Design review of the part built by this model. Coordinates are the model's own, in mm. A direction names the side the tool comes from. Coordinates: 2 decimals unless noted, no trailing zeros. Order: outer loops, then holes, each group sorted by start corner. A loop starts at its lowest first (then second) coordinate and runs counter-clockwise, first axis right, second up. Notation, with made-up numbers: M 82.5,15 L 101.5,15 A24 cw 101.5,25 Z; hole C -37,10.25 d7. An arc over 180 degrees is marked long. Answer as a JSON object with one key per item and string values.
Autodesk Inventor part; units mm, degrees
ref_plane "YZ Plane" through (0, 0, 0) normal (1, 0, 0) x (0, 1, 0)
ref_plane "XZ Plane" through (0, 0, 0) normal (0, 1, 0) x (-1, 0, 0)
ref_plane "XY Plane" through (0, 0, 0) normal (0, 0, 1) x (1, 0, 0)
sketch "Sketch1" plane through (0, 0, 0) normal (0, 1, 0) x (-1, 0, 0)
  point P0 (0, 0)
sketch "Sketch2" plane through (0, 0, 0) normal (0, 1, 0) x (-1, 0, 0)
  line L0 (0, 0) -> (40, 0)
  line L1 (40, 0) -> (40, -75)
  line L2 (40, -75) -> (0, -75)
  line L3 (0, -75) -> (0, -68)
  line L4 (0, -68) -> (27, -68)
  line L5 (35, -60) -> (35, -15)
  line L6 (27, -7) -> (0, -7)
  line L7 (0, -7) -> (0, 0)
  arc A0 (35, -15) -> (27, -7) centre (27, -15) ccw
  arc A1 (27, -68) -> (35, -60) centre (27, -60) ccw
  point P0 (35, -68)
  point P1 (35, -7)
  dimension "d0" = 40
  dimension "d1" = 75
  dimension "d2" = 40
  dimension "d3" = 7
  dimension "d5" = 35
  dimension "d6" = 61
  dimension "d7" = 8
extrude "Extrusion1" add sketch "Sketch2" along normal blind 500
properties part number "Channel2_CPY1"
1) Add section C-C (z = -36). State the section outline as (x, y) points.
Taken from the geometry:
{"outline": "M -40,0 L -35,0 L -35,500 L -40,500 Z"}
2) Add section B-B (y = 460). State the section outline as (x, z) points, and give its area (3 significant figures).
Taken from the geometry:
{"outline": "M -40,-75 L 0,-75 L 0,-68 L -27,-68 A8 cw -35,-60 L -35,-15 A8 cw -27,-7 L 0,-7 L 0,0 L -40,0 Z", "area": "892 mm2"}
3) To check wall thickness, follow L1, parallel to Z at x = -5, y = 85; L2, parallel to X at y = 54, z = -45; L3, parallel to Z at x = -30.5, y = 437. State the ranges of each line that lie inside material, in increasing order.
Taken from the geometry:
{"L1": "z = -75 to -68, -7 to 0", "L2": "x = -40 to -35", "L3": "z = -75 to -67.19, -7.81 to 0"}
4) Insertion check: pin 1 Ø1 at (y, z) = (56.5, -41.5) entering from +X; pin 2 Ø1 at (y, z) = (58.5, -9) entering from +X. Each pin has a flat end and moves straight along its axis. Give the tip position at first contact, or say it passes through.
Taken from the geometry:
{"pin 1": "stops at x = -35", "pin 2": "stops at x = -31.66"}
5) Add section A-A (x = -21.5). State the section outline as (y, z) points.
Taken from the geometry:
{"outline": "M 0,-75 L 500,-75 L 500,-68 L 0,-68 Z; M 0,-7 L 500,-7 L 500,0 L 0,0 Z"}
6) Mouldability with a two-part tool opening along Z and no side actions: class faces 3 (the flat face through (-35, 246, -38)), 4 (the flat face through (-20, 246, 0)), 5 (the flat face through (-36, 500, -32)) as released by +Z, released by -Z, zero draft, split by the parting line, or undercut.
Taken from the geometry:
{"face 3": "undercut", "face 4": "released by +Z", "face 5": "zero draft"}
7) Tool access review of faces 1 (the cylindrical face through (-32.594, 246.5, -9.281)), 2 (the flat face through (-36, 0, -32)): name each direction out of +Z, -Z, +X, -X, +Y, -Y from which nothing blocks a thin tool from reaching the whole face with its end or side.
Taken from the geometry:
{"face 1": "+X, +Y, -Y", "face 2": "+Z, -Z, +X, -X, -Y"}
